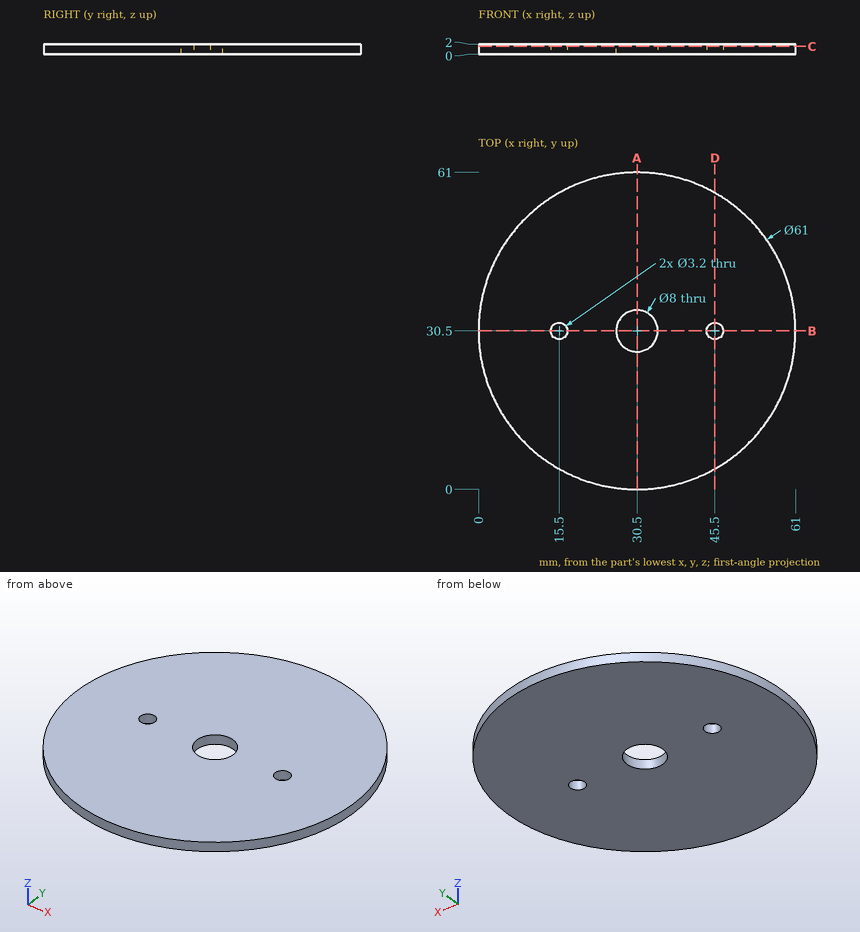
Can you work these out from the drawing? Everything is in mm from the part's minimum corner. Round coordinates to 2 decimals unless told otherwise and drop trailing zeros. Order: outer loops, then holes, each group sorted by start corner. A loop starts at its lowest first (then second) coordinate and runs counter-clockwise, first axis right, second up. Notation, with made-up numbers: (-23, 71) -> (-5, 71) arc R30 cw to (-5, 93) -> close; hole circle Ø6 at (39, 18). An arc over 180 degrees is marked (long way). Return JSON: item names as keys, results as strings. Group by question number.
1. If we section it at B-B, the plane y = 30.5: Write out the boundary of the cut face in (x, z), then the cut area to 3 significant figures.
2. If we section it at A-A, the plane x = 30.5: Write out the boundary of the cut face in (y, z), then the cut area to 3 significant figures.
3. I need wall thicknesses on line 1 (X direction, y = 29.5, z = 1.55); line 2 (Y direction, x = 15.5, z = 0.4); line 3 (Y direction, x = 30.5, z = 1.4). Which ranges of each line are inside material? Lowest first, please. Write a range as [from, to].
4. Will these pins go through, and if not, where does the flat tip stop? pin 1 (5 mm diameter, centred on x = 30.5, y = 30.5, fed in from +Z); pin 2 (10 mm diameter, centred on x = 38, y = 27, fed in from -Z).
5. If we section it at C-C, the plane z = 1.55: Write out the boundary of the cut face in (x, y), then the cut area to 3 significant figures.
6. If we section it at D-D, the plane x = 45.5: Write out the boundary of the cut face in (y, z).
Output values:
{
 "1": {"outline": "(0, 0) -> (13.9, 0) -> (13.9, 2) -> (0, 2) -> close; (17.1, 0) -> (26.5, 0) -> (26.5, 2) -> (17.1, 2) -> close; (34.5, 0) -> (43.9, 0) -> (43.9, 2) -> (34.5, 2) -> close; (47.1, 0) -> (61, 0) -> (61, 2) -> (47.1, 2) -> close", "area": "93.2 mm²"},
 "2": {"outline": "(0, 0) -> (26.5, 0) -> (26.5, 2) -> (0, 2) -> close; (34.5, 0) -> (61, 0) -> (61, 2) -> (34.5, 2) -> close", "area": "106 mm²"},
 "3": {"line 1": "[0.02, 14.25], [16.75, 26.63], [34.37, 44.25], [46.75, 60.98]", "line 2": "[3.94, 28.9], [32.1, 57.06]", "line 3": "[0, 26.5], [34.5, 61]"},
 "4": {"pin 1": "through", "pin 2": "z = 0"},
 "5": {"outline": "circle Ø61 at (30.5, 30.5); hole circle Ø3.2 at (15.5, 30.5); hole circle Ø8 at (30.5, 30.5); hole circle Ø3.2 at (45.5, 30.5)", "area": "2,860 mm²"},
 "6": {"outline": "(3.94, 0) -> (28.9, 0) -> (28.9, 2) -> (3.94, 2) -> close; (32.1, 0) -> (57.06, 0) -> (57.06, 2) -> (32.1, 2) -> close"}
}
